from build123d import *

# Parameters (mm, degrees)
SKETCH1_W             = 73.400000004
SKETCH1_H             = 64
BOSS_EXTRUDE1_DEPTH   = 4
BOSS_EXTRUDE2_DEPTH   = 4
SKETCH2_3_R           = 1.6
CUT_EXTRUDE1_DEPTH    = 4
BOSS_EXTRUDE3_DEPTH   = 4
SKETCH2_5_R           = 1.6
CUT_EXTRUDE2_DEPTH    = 4
SKETCH3_W             = 10
SKETCH3_H             = 4.5
BOSS_EXTRUDE4_DEPTH   = 4
BOSS_EXTRUDE4_2_DEPTH = 4
BOSS_EXTRUDE4_3_DEPTH = 4


with BuildPart() as part:
    # Sketch1 → Boss-Extrude1 (new body)
    with BuildSketch(Plane.XY):
        with Locations((0.200000002, -2.2)):
            Rectangle(SKETCH1_W, SKETCH1_H)
    extrude(amount=BOSS_EXTRUDE1_DEPTH)

    # Sketch2 → Boss-Extrude2 (add)
    with BuildSketch(Plane.XY.offset(4)):
        with BuildLine():
            ThreePointArc((21.433466103, -34.2), (24.9, -36.204218764), (28.366533897, -34.2))
            Line((28.366533897, -34.2), (21.433466103, -34.2))
        make_face()
    boss_extrude2 = extrude(amount=-BOSS_EXTRUDE2_DEPTH)

    # Sketch2<3> → Cut-Extrude1 (cut)
    with BuildSketch(Plane.XY.offset(4)):
        with Locations((24.9, -32.204218764)):
            Circle(SKETCH2_3_R)
    cut_extrude1 = extrude(amount=-CUT_EXTRUDE1_DEPTH, mode=Mode.SUBTRACT)

    # Mirror1: Boss-Extrude2, Cut-Extrude1 across plane
    add(boss_extrude2.mirror(Plane(origin=(0.200000002, 0, 0), x_dir=(0, 0, 1), z_dir=(1, 0, 0))))
    add(cut_extrude1.mirror(Plane(origin=(0.200000002, 0, 0), x_dir=(0, 0, 1), z_dir=(1, 0, 0))), mode=Mode.SUBTRACT)

    # Sketch2<4> → Boss-Extrude3 (add)
    with BuildSketch(Plane.XY.offset(4)):
        with BuildLine():
            ThreePointArc((-36.5, 23.264101615), (-38.5, 19.8), (-36.5, 16.335898385))
            Line((-36.5, 16.335898385), (-36.5, 23.264101615))
        make_face()
    boss_extrude3 = extrude(amount=-BOSS_EXTRUDE3_DEPTH)

    # Sketch2<5> → Cut-Extrude2 (cut)
    with BuildSketch(Plane.XY.offset(4)):
        with Locations((-34.5, 19.8)):
            Circle(SKETCH2_5_R)
    cut_extrude2 = extrude(amount=-CUT_EXTRUDE2_DEPTH, mode=Mode.SUBTRACT)

    # Mirror3: Boss-Extrude3, Cut-Extrude2 across plane
    add(boss_extrude3.mirror(Plane(origin=(0, -2.2, 0), x_dir=(0, 0, 1), z_dir=(0, -1, 0))))
    add(cut_extrude2.mirror(Plane(origin=(0, -2.2, 0), x_dir=(0, 0, 1), z_dir=(0, -1, 0))), mode=Mode.SUBTRACT)


with BuildPart() as body_2:
    # Sketch3 → Boss-Extrude4 (new body)
    with BuildSketch(Plane(origin=(0, 0, 0), x_dir=(-1, 0, 0), z_dir=(0, 0, -1))):
        with Locations((-20.200000004, 31.75)):
            Rectangle(SKETCH3_W, SKETCH3_H)
    extrude(amount=-BOSS_EXTRUDE4_DEPTH)


with BuildPart() as body_3:
    # Sketch3 → Boss-Extrude4 2 (new body)
    with BuildSketch(Plane(origin=(0, 0, 0), x_dir=(-1, 0, 0), z_dir=(0, 0, -1))):
        with Locations((-0.200000004, 31.75)):
            Rectangle(SKETCH3_W, SKETCH3_H)
    extrude(amount=-BOSS_EXTRUDE4_2_DEPTH)


with BuildPart() as body_4:
    # Sketch3 → Boss-Extrude4 3 (new body)
    with BuildSketch(Plane(origin=(0, 0, 0), x_dir=(-1, 0, 0), z_dir=(0, 0, -1))):
        with Locations((19.799999996, 31.75)):
            Rectangle(SKETCH3_W, SKETCH3_H)
    extrude(amount=-BOSS_EXTRUDE4_3_DEPTH)


with BuildPart() as body_2_1:
    add(body_2.part)

    # Combine1: union part, body 3, body 4
    add(part.part)
    add(body_3.part)
    add(body_4.part)


solid = body_2_1.part
For this review, take the finished solid that the model builds, in its own axes (mm). A direction names the side the tool comes from. Coordinates: 2 decimals unless noted, no trailing zeros. Loops run counter-clockwise (first coordinate to the right, second up) from the corner with the lowest first, then second, coordinate; pieces in that order, holes last. Notation, with made-up numbers: (49, 58) - (71, 58) arc R25 ccw to (71, 81) - close; hole circle Ø9 at (36, 38). An arc over 180 degrees is marked (long way). Use a Markdown table: item, result. Add a question column.
Item 1: Mouldability with a two-part tool opening along X and no side actions: class faces 4 (the face through (-24.8, 32, 2)), 5 (the face through (10, 29.8, 2)), 6 (the face through (33, -34.2, 2)) as pulls with the +X half, pulls with the -X half, needs draft (parallel to the pull), parting line crosses it, or undercut.
Item 2: We need section D-D (x = 2.5). Give the boundary of the cut face in (y, z), and give its area (3 significant figures).
Item 3: For line 1 (Y direction, x = -34.5, z = 0.9); line 2 (X direction, y = -32, z = 1.5); line 3 (X direction, y = -24, z = 0.7) (3 decimals), list the stretches that pass through material, from the lowest coordinate up.
Item 4: We need section C-C (z = 2.6). Give the boundary of the cut face in (x, y), and give its area (3 significant figures).
Item 5: We need section A-A (y = 19.8). Give the boundary of the cut face in (x, z), and give its area (3 significant figures).
Item 6: Insertion check: pin 1 Ø2 at (x, z) = (23.5, 2) entering from -Y; pin 2 Ø1.2 at (x, z) = (-31, 2.5) entering from -Y; pin 3 Ø1.5 at (y, z) = (21, 3.5) entering from -X; pin 4 Ø5 at (x, y) = (-28.5, -14.5) entering from -Z. Each pin has a flat end and moves straight along its axis. Give the tip position at first contact, or say it passes through.
Item 7: We need section B-B (x = -34.5). Give the boundary of the cut face in (y, z).
Item 8: Tool access review of faces 1 (the face through (-32, -34.2, 2)), 2 (the face through (-31, 29.8, 2)), 3 (the face through (5.2, 32, 2)): name each direction out of +Z, -Z, +X, -X, +Y, -Y from which nothing blocks a thin tool from reaching the whole face with its end or side.
Results list:
| question | item | result |
|---|---|---|
| 1 | face 4 | pulls with the -X half |
| 1 | face 5 | undercut |
| 1 | face 6 | needs draft |
| 2 | outline | (-34.2, 0) - (34, 0) - (34, 4) - (-34.2, 4) - close |
| 2 | area | 273 mm^2 |
| 3 | line 1 | y = -34.2 to -25.8, -22.6 to 18.2, 21.4 to 29.8 |
| 3 | line 2 | x = -36.5 to -26.09, -22.91 to 23.31, 26.49 to 36.9 |
| 3 | line 3 | x = -38.495 to -36.087, -32.913 to 36.9 |
| 4 | outline | (-36.5, -34.2) - (-27.97, -34.2) arc R4 ccw to (-21.03, -34.2) - (21.43, -34.2) arc R4 ccw to (28.37, -34.2) - (36.9, -34.2) - (36.9, 29.8) - (25.2, 29.8) - (25.2, 34) - (15.2, 34) - (15.2, 29.8) - (5.2, 29.8) - (5.2, 34) - (-4.8, 34) - (-4.8, 29.8) - (-14.8, 29.8) - (-14.8, 34) - (-24.8, 34) - (-24.8, 29.8) - (-36.5, 29.8) - (-36.5, 23.26) arc R4 ccw to (-36.5, 16.34) - (-36.5, -20.74) arc R4 ccw to (-36.5, -27.66) - close; hole circle Ø3.2 at (-34.5, -24.2); hole circle Ø3.2 at (-34.5, 19.8); hole circle Ø3.2 at (-24.5, -32.2); hole circle Ø3.2 at (24.9, -32.2) |
| 4 | area | 4,830 mm^2 |
| 5 | outline | (-38.5, 0) - (-36.1, 0) - (-36.1, 4) - (-38.5, 4) - close; (-32.9, 0) - (36.9, 0) - (36.9, 4) - (-32.9, 4) - close |
| 5 | area | 289 mm^2 |
| 6 | pin 1 | stops at y = -36.18 |
| 6 | pin 2 | stops at y = -34.2 |
| 6 | pin 3 | stops at x = -38.47 |
| 6 | pin 4 | stops at z = 0 |
| 7 | outline | (-34.2, 0) - (-25.8, 0) - (-25.8, 4) - (-34.2, 4) - close; (-22.6, 0) - (18.2, 0) - (18.2, 4) - (-22.6, 4) - close; (21.4, 0) - (29.8, 0) - (29.8, 4) - (21.4, 4) - close |
| 8 | face 1 | +Z, -Z, -X, -Y |
| 8 | face 2 | +Z, -Z, -X, +Y |
| 8 | face 3 | +Z, -Z, +Y |
